from build123d import *

# Parameters (mm, degrees)
F0_R     = 5.7785
F1_DEPTH = 12.7
F2_R     = 5.08
F3_DEPTH = 2.3622
F5_DEPTH = 7.0104
F7_DEPTH = 12.7
F8_R     = 0.79375
F9_DEPTH = 7.7978


with BuildPart() as f1:
    # F0 (on Top) → F1 (new body)
    with BuildSketch(Plane.XY):
        Circle(F0_R)
    extrude(amount=F1_DEPTH)

    # F2 (on face) → F3 (cut)
    with BuildSketch(Plane(origin=(0, 0, 0), x_dir=(1, 0, 0), z_dir=(0, 0, -1))):
        Circle(F2_R)
    extrude(amount=-F3_DEPTH, mode=Mode.SUBTRACT)

    # F4 (on face) → F5 (cut)
    with BuildSketch(Plane(origin=(0, 0, 2.3622), x_dir=(1, 0, 0), z_dir=(0, 0, -1))):
        with BuildLine():
            Line((2.3622, -2.0447), (2.3622, 2.0447))
            ThreePointArc((2.3622, 2.0447), (1.670328, 3.715028), (0, 4.4069))
            ThreePointArc((0, 4.4069), (-1.670328, 3.715028), (-2.3622, 2.0447))
            Line((-2.3622, 2.0447), (-2.3622, -2.0447))
            ThreePointArc((-2.3622, -2.0447), (-1.670328, -3.715028), (0, -4.4069))
            ThreePointArc((0, -4.4069), (1.670328, -3.715028), (2.3622, -2.0447))
        make_face()
    extrude(amount=-F5_DEPTH, mode=Mode.SUBTRACT)

    # F6 (on Right) → F7 (cut, symmetric)
    with BuildSketch(Plane.YZ):
        with BuildLine():
            ThreePointArc((0, 4.6355), (0.835164, 4.981436), (1.1811, 5.8166))
            ThreePointArc((1.1811, 5.8166), (-0.835164, 6.651764), (0, 4.6355))
        make_face()
    extrude(amount=F7_DEPTH, both=True, mode=Mode.SUBTRACT)

    # F8 (on face) → F9 (join)
    with BuildSketch(Plane.XY.offset(12.7)):
        Circle(F8_R)
    extrude(amount=F9_DEPTH)


solid = f1.part
The listing builds one solid part. Answer for the finished solid, in the listing's coordinates (mm). A direction names the side the tool comes from. Give positions to 0.01 mm unless a question says otherwise; leave off trailing zeros. Order: outer loops, then holes, each group sorted by start corner. A loop starts at its lowest first (then second) coordinate and runs counter-clockwise, first axis right, second up. Notation, with made-up numbers: (-6, -26) - (1, -26) arc R26 cw to (1, -5) - close; hole circle Ø5 at (17, 68.25). An arc over 180 degrees is marked (long way). One line per item, written item: value. Start each with the question number.
1) The mould has two halves that part along Y. Classify faces 3 (the face through (-0.661, -5.037, 1.165)), 4 (the face through (1, 0, 12.7)), 5 (the face through (-0.172, -0.775, 16.544)): released by +Y, released by -Y, zero draft, split by the parting line, or undercut.
2) A tool of negligible diameter and unlimited length cuts with its end or side. For faces 1 (the face through (5.51, 1.74, 6.26)), 2 (the face through (2.362, 1, 7)), from which of +Z, -Z, +X, -X, +Y, -Y can it reach the whole face along a straight path? Write none if from no direction.
3) A cutting plane is placed at B-B on x = -3.75. Give the vertices of the cut face in (y, z), then the cut area to 3 significant figures.
4) A cutting plane is placed at A-A on z = 7.5. Give the vertices of the cut face in (x, y), then the cut area to 3 significant figures.
5) Given pin 1 Ø1 at (x, y) = (-1, -0.5) entering from -Z; pin 2 Ø6 at (x, z) = (-1.5, 16) entering from +Y; pin 3 Ø3 at (x, y) = (-2, 1.5) entering from -Z, each flat-ended and moving along its own axis, determine where each tip first touches the part or whether it passes through.
6) Find the intervals of material crossed by L1, parallel to Z at x = 4.85, y = 0; L2, parallel to Y at x = 0, z = 1.5; L3, parallel to Z at x = -1.5, y = -4.25, in increasing order.
7) A cutting plane is placed at C-C on y = -3.5. Give the vertices of the cut face in (x, z), then the cut area to 3 significant figures.
8) A cutting plane is placed at D-D on x = -1.5. Give the vertices of the cut face in (y, z), then the cut area to 3 significant figures.
Answer sheet:
1. face 3: undercut
1. face 4: zero draft
1. face 5: split by the parting line
2. face 1: +Z, -Z
2. face 2: -Z
3. outline: (-4.4, 0) - (-3.43, 0) - (-3.43, 2.36) - (3.43, 2.36) - (3.43, 0) - (4.4, 0) - (4.4, 12.7) - (-4.4, 12.7) - close; hole circle Ø2.36 at (0, 5.82)
3. area: 91.1 mm2
4. outline: circle Ø11.56 at (0, 0); hole (-2.36, -2.04) arc R2.36 ccw to (0, -4.41) arc R2.36 ccw to (2.36, -2.04) - (2.36, 2.04) arc R2.36 ccw to (0, 4.41) arc R2.36 ccw to (-2.36, 2.04) - close
4. area: 68.1 mm2
5. pin 1: stops at z = 9.37
5. pin 2: stops at y = 0.79
5. pin 3: stops at z = 2.36
6. L1: z = 2.36 to 4.64, 7 to 12.7
6. L2: y = -5.78 to -5.08, 5.08 to 5.78
6. L3: z = 2.36 to 12.7
7. outline: (-4.6, 0) - (-3.68, 0) - (-3.68, 2.36) - (-1.86, 2.36) - (-1.86, 9.37) - (1.86, 9.37) - (1.86, 2.36) - (3.68, 2.36) - (3.68, 0) - (4.6, 0) - (4.6, 12.7) - (-4.6, 12.7) - close
7. area: 73.3 mm2
8. outline: (-5.58, 0) - (-4.85, 0) - (-4.85, 2.36) - (-3.87, 2.36) - (-3.87, 9.37) - (3.87, 9.37) - (3.87, 2.36) - (4.85, 2.36) - (4.85, 0) - (5.58, 0) - (5.58, 12.7) - (-5.58, 12.7) - close
8. area: 64.6 mm2
